Geometry check sheet. Reference: the model listing, model coordinates, mm. Give positions to 0.01 mm unless a question says otherwise; leave off trailing zeros. Loops run counter-clockwise (first coordinate to the right, second up) from the corner with the lowest first, then second, coordinate; pieces in that order, holes last.
1. Go/stop test with a flat-tipped pin: pin 1 Ø16 at (x, y) = (120.83, 34.13) entering from +Z. Record where the tip stops, or that it passes through.
2. Cross-section at C-C, the plane y = 31. State how many separate pieces and enclosed holes the cut face has, plus the area to 3 significant figures.
3. Cross-section at B-B, the plane x = 195. Record the cut outline in (y, z) (3 decimals), plus the area to 3 significant figures.
4. Material ranges on L1, parallel to Y at x = 139.5, z = 1.5; L2, parallel to Y at x = 248, z = 2.3, recorded low to high.
5. Cross-section at A-A, the plane x = 224. Record the cut outline in (y, z) (3 decimals).
6. Release check for a two-part mould opening along X. For faces 1 (the cylindrical face through (10.224, 63.423, 1.61)), 2 (the flat face through (128, 27, 0)), 3 (the cylindrical face through (179.13, 54.88, 1.61)) record: +X half, -X half, draft (parallel to the pull), parting line (faces both ways), or undercut.
from build123d import *

# Parameters (mm, degrees)
F0_W     = 260.35
F0_H     = 68.2625
F1_DEPTH = 3.175
F2_W     = 6.35
F2_H     = 2.38125
F2_R     = 9.017
F3_DEPTH = 3.175
F4_W     = 3.175
F4_H     = 3.175
F5_DEPTH = 260.35


with BuildPart() as f1:
    # F0 (on Top) → F1 (new body)
    with BuildSketch(Plane.XY):
        with Locations((130.175, 34.13125)):
            Rectangle(F0_W, F0_H)
    extrude(amount=F1_DEPTH)

    # F2 (on face) → F3 (cut, through all)
    with BuildSketch(Plane.XY.offset(3.175)):
        with Locations((3.175, 1.190625)):
            Rectangle(F2_W, F2_H)
        with Locations((3.175, 67.071875)):
            Rectangle(F2_W, F2_H)
        with Locations((11.39825, 54.483)):
            Circle(F2_R)
        with Locations((31.668861, 54.483)):
            Circle(F2_R)
        with Locations((51.939472, 54.483)):
            Circle(F2_R)
        with Locations((72.210083, 54.483)):
            Circle(F2_R)
        with Locations((101.356583, 54.483)):
            Circle(F2_R)
        with Locations((121.627194, 54.483)):
            Circle(F2_R)
        with Locations((140.310306, 54.483)):
            Circle(F2_R)
        with Locations((158.993417, 54.483)):
            Circle(F2_R)
        with Locations((188.139917, 54.483)):
            Circle(F2_R)
        with Locations((208.410528, 54.483)):
            Circle(F2_R)
        with Locations((228.681139, 54.483)):
            Circle(F2_R)
        with Locations((248.95175, 54.483)):
            Circle(F2_R)
        with Locations((11.39825, 34.13125)):
            Circle(F2_R)
        with Locations((31.668861, 34.13125)):
            Circle(F2_R)
        with Locations((51.939472, 34.13125)):
            Circle(F2_R)
        with Locations((72.210083, 34.13125)):
            Circle(F2_R)
        with Locations((248.95175, 34.13125)):
            Circle(F2_R)
        with Locations((228.681139, 34.13125)):
            Circle(F2_R)
        with Locations((208.410528, 34.13125)):
            Circle(F2_R)
        with Locations((188.139917, 34.13125)):
            Circle(F2_R)
        with Locations((102.150333, 34.13125)):
            Circle(F2_R)
        with Locations((120.833444, 34.13125)):
            Circle(F2_R)
        with Locations((139.516556, 34.13125)):
            Circle(F2_R)
        with Locations((158.199667, 34.13125)):
            Circle(F2_R)
        with Locations((11.39825, 13.7795)):
            Circle(F2_R)
        with Locations((248.95175, 13.7795)):
            Circle(F2_R)
        with Locations((228.681139, 13.7795)):
            Circle(F2_R)
        with Locations((208.410528, 13.7795)):
            Circle(F2_R)
        with Locations((188.139917, 13.7795)):
            Circle(F2_R)
        with Locations((31.668861, 13.7795)):
            Circle(F2_R)
        with Locations((51.939472, 13.7795)):
            Circle(F2_R)
        with Locations((72.210083, 13.7795)):
            Circle(F2_R)
        with Locations((102.150333, 13.7795)):
            Circle(F2_R)
        with Locations((120.833444, 13.7795)):
            Circle(F2_R)
        with Locations((139.516556, 13.7795)):
            Circle(F2_R)
        with Locations((158.199667, 13.7795)):
            Circle(F2_R)
        with Locations((15.875, 67.071875)):
            Rectangle(F2_W, F2_H)
        with Locations((15.875, 1.190625)):
            Rectangle(F2_W, F2_H)
        with Locations((28.575, 1.190625)):
            Rectangle(F2_W, F2_H)
        with Locations((41.275, 1.190625)):
            Rectangle(F2_W, F2_H)
        with Locations((53.975, 1.190625)):
            Rectangle(F2_W, F2_H)
        with Locations((66.675, 1.190625)):
            Rectangle(F2_W, F2_H)
        with Locations((79.375, 1.190625)):
            Rectangle(F2_W, F2_H)
        with Locations((92.075, 1.190625)):
            Rectangle(F2_W, F2_H)
        with Locations((104.775, 1.190625)):
            Rectangle(F2_W, F2_H)
        with Locations((117.475, 1.190625)):
            Rectangle(F2_W, F2_H)
        with Locations((130.175, 1.190625)):
            Rectangle(F2_W, F2_H)
        with Locations((142.875, 1.190625)):
            Rectangle(F2_W, F2_H)
        with Locations((155.575, 1.190625)):
            Rectangle(F2_W, F2_H)
        with Locations((168.275, 1.190625)):
            Rectangle(F2_W, F2_H)
        with Locations((180.975, 1.190625)):
            Rectangle(F2_W, F2_H)
        with Locations((193.675, 1.190625)):
            Rectangle(F2_W, F2_H)
        with Locations((206.375, 1.190625)):
            Rectangle(F2_W, F2_H)
        with Locations((219.075, 1.190625)):
            Rectangle(F2_W, F2_H)
        with Locations((231.775, 1.190625)):
            Rectangle(F2_W, F2_H)
        with Locations((244.475, 1.190625)):
            Rectangle(F2_W, F2_H)
        with Locations((257.175, 1.190625)):
            Rectangle(F2_W, F2_H)
        with Locations((269.875, 1.190625)):
            Rectangle(F2_W, F2_H)
        with Locations((282.575, 1.190625)):
            Rectangle(F2_W, F2_H)
        with Locations((28.575, 67.071875)):
            Rectangle(F2_W, F2_H)
        with Locations((41.275, 67.071875)):
            Rectangle(F2_W, F2_H)
        with Locations((53.975, 67.071875)):
            Rectangle(F2_W, F2_H)
        with Locations((66.675, 67.071875)):
            Rectangle(F2_W, F2_H)
        with Locations((79.375, 67.071875)):
            Rectangle(F2_W, F2_H)
        with Locations((92.075, 67.071875)):
            Rectangle(F2_W, F2_H)
        with Locations((104.775, 67.071875)):
            Rectangle(F2_W, F2_H)
        with Locations((117.475, 67.071875)):
            Rectangle(F2_W, F2_H)
        with Locations((130.175, 67.071875)):
            Rectangle(F2_W, F2_H)
        with Locations((142.875, 67.071875)):
            Rectangle(F2_W, F2_H)
        with Locations((155.575, 67.071875)):
            Rectangle(F2_W, F2_H)
        with Locations((168.275, 67.071875)):
            Rectangle(F2_W, F2_H)
        with Locations((180.975, 67.071875)):
            Rectangle(F2_W, F2_H)
        with Locations((193.675, 67.071875)):
            Rectangle(F2_W, F2_H)
        with Locations((206.375, 67.071875)):
            Rectangle(F2_W, F2_H)
        with Locations((219.075, 67.071875)):
            Rectangle(F2_W, F2_H)
        with Locations((231.775, 67.071875)):
            Rectangle(F2_W, F2_H)
        with Locations((244.475, 67.071875)):
            Rectangle(F2_W, F2_H)
        with Locations((257.175, 67.071875)):
            Rectangle(F2_W, F2_H)
        with Locations((269.875, 67.071875)):
            Rectangle(F2_W, F2_H)
        with Locations((282.575, 67.071875)):
            Rectangle(F2_W, F2_H)
    extrude(amount=-F3_DEPTH, mode=Mode.SUBTRACT)

    # F4 (on face) → F5 (join, through all)
    with BuildSketch(Plane(origin=(0, 0, 0), x_dir=(0, -1, 0), z_dir=(-1, 0, 0))):
        with Locations((-0.79375, 1.5875)):
            Rectangle(F4_W, F4_H)
        with Locations((-67.46875, 1.5875)):
            Rectangle(F4_W, F4_H)
    extrude(amount=-F5_DEPTH)


solid = f1.part
Result:
1. pin 1: passes through
2. separate pieces: 13
2. enclosed holes: 0
2. area: 182 mm2
3. outline: (-0.794, 0) - (7.928, 0) - (7.928, 3.175) - (-0.794, 3.175) - close; (19.631, 0) - (28.279, 0) - (28.279, 3.175) - (19.631, 3.175) - close; (39.983, 0) - (48.631, 0) - (48.631, 3.175) - (39.983, 3.175) - close; (60.335, 0) - (69.056, 0) - (69.056, 3.175) - (60.335, 3.175) - close
3. area: 110 mm2
4. L1: y = -0.79 to 4.76, 22.8 to 25.11, 43.15 to 45.5, 63.46 to 69.06
4. L2: y = -0.79 to 4.81, 22.75 to 25.16, 43.1 to 45.52, 63.45 to 69.06
5. outline: (-0.794, 0) - (6.073, 0) - (6.073, 3.175) - (-0.794, 3.175) - close; (21.486, 0) - (26.425, 0) - (26.425, 3.175) - (21.486, 3.175) - close; (41.838, 0) - (46.776, 0) - (46.776, 3.175) - (41.838, 3.175) - close; (62.19, 0) - (69.056, 0) - (69.056, 3.175) - (62.19, 3.175) - close
6. face 1: undercut
6. face 2: draft
6. face 3: undercut
